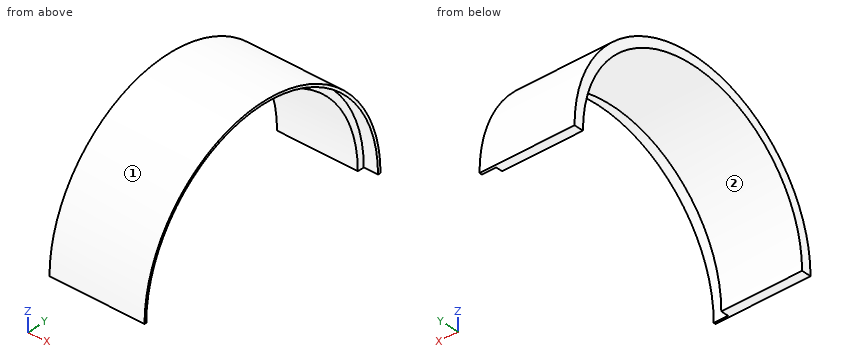
```python
from build123d import *

# Parameters (mm, degrees)
BOSS_EXTRUDE1_DEPTH = 508
CAVITY1_START       = 431.8
CAVITY1_DEPTH       = 76.2


# Read off the part's stored shape, not the designer's step: Cavity1
with BuildPart() as part:
    # Sketch1 → Boss-Extrude1 (new body)
    with BuildSketch(Plane(origin=(0, 0, 0), x_dir=(0, 0, -1), z_dir=(1, 0, 0))):
        with BuildLine():
            Line((0, 711.2), (0, 660.4))
            ThreePointArc((0, 660.4), (-660.4, 0), (0, -660.4))
            Line((0, -660.4), (0, -711.2))
            ThreePointArc((0, -711.2), (-711.2, 0), (0, 711.2))
        make_face()
    extrude(amount=BOSS_EXTRUDE1_DEPTH)

    # Cavity1 outline → Cavity1 (cut)
    with BuildSketch(Plane.YZ.offset(CAVITY1_START)):
        with BuildLine():
            ThreePointArc((696.250142702, 0), (-2.249857298, 698.5), (-700.749857298, 0))
            Line((-700.749857298, 0), (-660.4, 0))
            ThreePointArc((-660.4, 0), (0, 660.4), (660.4, 0))
            Line((660.4, 0), (696.250142702, 0))
        make_face()
    extrude(amount=CAVITY1_DEPTH, mode=Mode.SUBTRACT)


solid = part.part
```
Source: CAD feature listing. Evaluate the final solid. Frame: model axes, mm. Face numbers are marked on the shaded views. Give positions to 0.01 mm unless a question says otherwise; leave off trailing zeros. Write each loop counter-clockwise with the first axis right and the second up, starting at its lowest first coordinate (ties: lowest second). Pieces come first, ordered by that corner, then holes. Notation, with made-up numbers: (0.5, 40.5) - (40.5, 40.5) arc R14 ccw to (40.5, 62.5) - close; hole circle Ø2 at (2.5, 28). An arc over 180 degrees is marked (long way). One line per item, written item: value. Start each with the question number.
Q1. Section query A-A, the plane z = 146.5. Return the cut outline in (x, y), then the cut area to 3 significant figures.
Q2. First-contact query: pin 1 Ø5 at (x, y) = (327, 519) entering from +Z; pin 2 Ø8 at (x, y) = (73.5, 203) entering from +Z; pin 3 Ø1 at (x, z) = (183.5, 342) entering from +Y. Flat tips, straight axial feed; report the tip coordinate or a pass-through.
Q3. Draft query along Y for the marked faces 1 and 2. Return one class per face: +Y half, -Y half, draft (parallel to the pull), parting line (faces both ways), or undercut.
Q4. Section query C-C, the plane z = 73. Return the cut outline in (x, y), then the cut area to 3 significant figures.
Q5. Section query D-D, the plane x = 322. Return the cut outline in (y, z).
Q6. Material intervals for probe 1 along Y at (x, z) = (222, 36.5); probe 2 along Z at (x, y) = (445, -12.5); probe 3 along Y at (x, z) = (338, 608), sorted ascending. Write a range as from..to.
Q7. Section query B-B, the plane y = -482. Return the cut outline in (x, z).
Answer:
1. outline: (0, -695.95) - (508, -695.95) - (508, -685.21) - (431.8, -685.21) - (431.8, -643.95) - (0, -643.95) - close; (0, 643.95) - (431.8, 643.95) - (431.8, 680.71) - (508, 680.71) - (508, 695.95) - (0, 695.95) - close
1. area: 46,900 mm2
2. pin 1: stops at z = 488.91
2. pin 2: stops at z = 682.79
2. pin 3: stops at y = 623.85
3. face 1: parting line
3. face 2: undercut
4. outline: (0, -707.44) - (508, -707.44) - (508, -696.92) - (431.8, -696.92) - (431.8, -656.35) - (0, -656.35) - close; (0, 656.35) - (431.8, 656.35) - (431.8, 692.43) - (508, 692.43) - (508, 707.44) - (0, 707.44) - close
4. area: 46,100 mm2
5. outline: (-711.2, 0) - (-660.4, 0) arc R660.4 cw to (660.4, 0) - (711.2, 0) arc R711.2 ccw to start
6. probe 1: y = -710.26..-659.39, 659.39..710.26
6. probe 2: z = 698.42..711.09
6. probe 3: y = -368.97..-257.81, 257.81..368.97
7. outline: (0, 451.45) - (431.8, 451.45) - (431.8, 507.68) - (508, 507.68) - (508, 522.95) - (0, 522.95) - close
